```python
from build123d import *

# Parameters (mm, degrees)
BOSS_EXTRUDE1_DEPTH     = 5
SKETCH2_R               = 1.25
CUT_EXTRUDE2_DEPTH      = 56.014202712
CUT_EXTRUDE3_DEPTH      = 56.014202712
CUT_EXTRUDE3_DEPTH_BACK = 56.014202712
SKETCH6_W               = 11
SKETCH6_H               = 4
SKETCH8_W               = 3
SKETCH8_H               = 2
BOSS_EXTRUDE4_DEPTH     = 47.5
SKETCH9_W               = 22.5
SKETCH9_H               = 3
CUT_EXTRUDE5_DEPTH      = 48.5


with BuildPart() as part:
    # Sketch1 → Boss-Extrude1 (new body)
    with BuildSketch(Plane(origin=(0, 0, 0), x_dir=(1, 0, 0), z_dir=(0, 1, 0))):
        Polygon((0, 0), (15, 0), (15, 35), (31.25, 35), (31.25, 45), (-16.25, 45), (-16.25, 35), (0, 35), align=None)
    extrude(amount=BOSS_EXTRUDE1_DEPTH)

    # Sketch2 → Cut-Extrude2 (cut, through all)
    with BuildSketch(Plane(origin=(15, 0, 0), x_dir=(0, 0, -1), z_dir=(1, 0, 0))):
        with Locations((3, 2.5)):
            Circle(SKETCH2_R)
    extrude(amount=-CUT_EXTRUDE2_DEPTH, mode=Mode.SUBTRACT)

    # Sketch6 → Cut-Extrude3 (cut, two sides: drawn at the far end of the back side and taken through both)
    with BuildSketch(Plane.XZ.offset(-CUT_EXTRUDE3_DEPTH_BACK)):
        with Locations((7.5, -30.5)):
            Rectangle(SKETCH6_W, SKETCH6_H)
    extrude(amount=CUT_EXTRUDE3_DEPTH + CUT_EXTRUDE3_DEPTH_BACK, mode=Mode.SUBTRACT)

    # Sketch8 → Boss-Extrude4 (add)
    with BuildSketch(Plane(origin=(31.25, 0, 0), x_dir=(0, 0, -1), z_dir=(1, 0, 0))):
        with Locations((40.5, 6)):
            Rectangle(SKETCH8_W, SKETCH8_H)
        Polygon((34.5, 8), (32.5, 8), (32.5, 0), (35, 0), (35, 5), (34.5, 5), align=None)
    extrude(amount=-BOSS_EXTRUDE4_DEPTH)

    # Sketch9 → Cut-Extrude5 (cut)
    with BuildSketch(Plane.XY.offset(-32.5)):
        with Locations((7.5, 6.5)):
            Rectangle(SKETCH9_W, SKETCH9_H)
    extrude(amount=-CUT_EXTRUDE5_DEPTH, mode=Mode.SUBTRACT)


solid = part.part
```
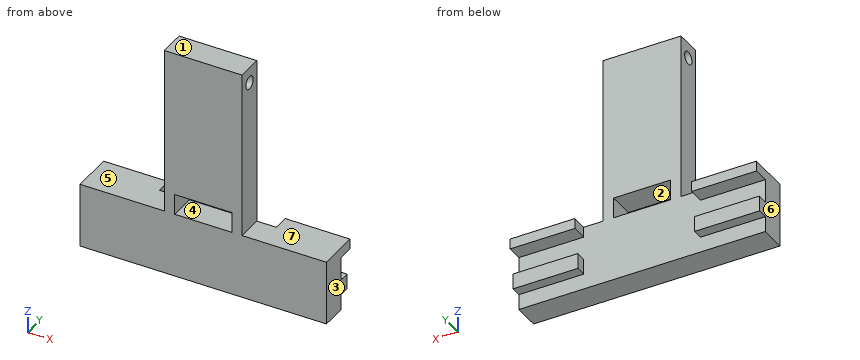
CAD build for the part. Positions are in the model's coordinates, mm. Face numbers are marked on the shaded views. A direction names the side the tool comes from. Round coordinates to 2 decimals unless told otherwise and drop trailing zeros. Order: outer loops, then holes, each group sorted by start corner. A loop starts at its lowest first (then second) coordinate and runs counter-clockwise, first axis right, second up.
Q1. Which spindle directions (+Z, -Z, +X, -X, +Y, -Y) get a long thin tool onto all of the face, cutting with end or side? Do the marked faces 5, 6 and 7. Say none if no direction does.
Q2. Slice it at C-C (z = -3). Write the cut outline in (x, y).
Q3. Wall check: L1, parallel to Y at x = 10, z = -3; L2, parallel to Y at x = 5, z = -38.5; L3, parallel to X at y = 1.25, z = -27. Give the ranges that are in metal, low to high.
Q4. Slice it at B-B (x = 5). Write the cut outline in (y, z).
Q5. Slice it at D-D (x = -10). Write the cut outline in (y, z).
Q6. Slice it at A-A (y = 2.5). Write the cut outline in (x, z).
Q7. Two-plate mould, pull along X, no slides. Class the marked faces 1, 2, 3 and 4: pulls with the +X half, pulls with the -X half, needs draft (parallel to the pull), parting line crosses it, or undercut.
Q8. Drop flat-ended pins along their axis: pin 1 (1.6 mm diameter, centred on x = 27.5, y = 5.5, fed in from -Z); pin 2 (1.5 mm diameter, centred on x = -10.5, z = -41, fed in from +Y); pin 3 (2 mm diameter, centred on x = -10.5, y = 7, fed in from -Z); pin 4 (2 mm diameter, centred on x = 21.5, y = 3.5, fed in from +Z). Give the stop position or say it passes through.
Results below:
1. face 5: +Z, -X, +Y, -Y
1. face 6: +Z, -Z, -X, +Y, -Y
1. face 7: +Z, +X, +Y, -Y
2. outline: (0, 0) - (15, 0) - (15, 1.25) - (0, 1.25) - close; (0, 3.75) - (15, 3.75) - (15, 5) - (0, 5) - close
3. L1: y = 0 to 1.25, 3.75 to 5
3. L2: y = 0 to 5
3. L3: x = 0 to 15
4. outline: (0, -45) - (5, -45) - (5, -32.5) - (0, -32.5) - close; (0, -28.5) - (5, -28.5) - (5, 0) - (0, 0) - close; hole circle Ø2.5 at (2.5, -3)
5. outline: (0, -45) - (5, -45) - (5, -42) - (7, -42) - (7, -39) - (5, -39) - (5, -34.5) - (8, -34.5) - (8, -32.5) - (0, -32.5) - close
6. outline: (-16.25, -45) - (31.25, -45) - (31.25, -32.5) - (15, -32.5) - (15, -4.25) - (0, -4.25) - (0, -32.5) - (-16.25, -32.5) - close; (0, -1.75) - (15, -1.75) - (15, 0) - (0, 0) - close; hole (2, -32.5) - (13, -32.5) - (13, -28.5) - (2, -28.5) - close
7. face 1: needs draft
7. face 2: undercut
7. face 3: pulls with the +X half
7. face 4: undercut
8. pin 1: stops at z = -45
8. pin 2: stops at y = 7
8. pin 3: stops at z = -42
8. pin 4: stops at z = -32.5
